```python
from build123d import *

# Parameters (mm, degrees)
F1_R     = 8.89
F1_R_2   = 5.9436
F3_R     = 8.89
F3_R_2   = 7.62
F4_DEPTH = 12.7
F5_R     = 8.89
F5_R_2   = 7.62
F6_DEPTH = 12.7


with BuildPart() as f2:
    # F2: sweep along a path in F0
    with BuildLine(Plane.XY) as f2_path:
        Line((0, 0), (0, 145.0086))
    # F1 (on Front) → F2 (sweep)
    with BuildSketch(Plane.XZ):
        Circle(F1_R)
        Circle(F1_R_2, mode=Mode.SUBTRACT)
    sweep(path=f2_path.line)

    # F3 (on face) → F4 (cut)
    with BuildSketch(Plane(origin=(0, 145.0086, 0), x_dir=(-1, 0, 0), z_dir=(0, 1, 0))):
        Circle(F3_R)
        Circle(F3_R_2, mode=Mode.SUBTRACT)
    extrude(amount=-F4_DEPTH, mode=Mode.SUBTRACT)

    # F5 (on face) → F6 (cut)
    with BuildSketch(Plane.XZ):
        Circle(F5_R)
        Circle(F5_R_2, mode=Mode.SUBTRACT)
    extrude(amount=-F6_DEPTH, mode=Mode.SUBTRACT)


solid = f2.part
```
The listing builds one solid part. Answer for the finished solid, in the listing's coordinates (mm). A direction names the side the tool comes from. Coordinates: 2 decimals unless noted, no trailing zeros. Write each loop counter-clockwise with the first axis right and the second up, starting at its lowest first coordinate (ties: lowest second). Pieces come first, ordered by that corner, then holes. Notation, with made-up numbers: (-35, 50.5) -> (-16, 50.5) arc R8 ccw to (-16, 64.5) -> close; hole circle Ø8 at (73.5, 44.25). An arc over 180 degrees is marked (long way). Write each question's results on one line, items separated by ' | '. Start each with the question number.
1) Flat-ended cylindrical pins translate along their axes: pin 1 Ø3 at (y, z) = (93.5, -4.5) entering from +X; pin 2 Ø8 at (y, z) = (18, -5.5) entering from +X; pin 3 Ø1 at (x, y) = (-5.5, 62.5) entering from -Z. Find the tip coordinate at first contact, or state that the pin passes through.
2) For a pull along X with two mould halves and no side action, classify faces 4 (the flat face through (-4, 0, 5)), 5 (the cylindrical face through (-1.93, 73.34, 8.68)), 6 (the cylindrical face through (5.669, 73.519, -1.785)) as +X half, -X half, draft (parallel to the pull), parting line (faces both ways), or undercut.
3) Straight lines are drawn through the part: probe 1 along Z at (x, y) = (0, 41.5); probe 2 along X at (y, z) = (138.5, -0.5); probe 3 along Z at (x, y) = (1.5, 33). For each, find the intervals that lie inside material, in ascending order.
4) A cutting plane is placed at B-B (z = 0). Determine the outline of the cut face in (x, y), then the cut area to 3 significant figures.
5) A cutting plane is placed at A-A (x = 0). Determine the outline of the cut face in (y, z), then the cut area to 3 significant figures.
6) A tool of negligible diameter and unlimited length cuts with its end or side. For faces 1 (the flat face through (-7, 132.309, 4)), 2 (the flat face through (-4, 145.009, 5)), 3 (the cylindrical face through (-1.65, 6.26, -7.44)), from which of +Z, -Z, +X, -X, +Y, -Y can it reach the whole face along a straight path? Write none if from no direction.
7) A cutting plane is placed at C-C (y = 130.5). Determine the outline of the cut face in (x, z), then the cut area to 3 significant figures.
Values follow:
1) pin 1: x = 8.37 | pin 2: x = 8.76 | pin 3: z = -7.35
2) face 4: draft | face 5: parting line | face 6: undercut
3) probe 1: -8.89 to -5.94, 5.94 to 8.89 | probe 2: -7.6 to -5.92, 5.92 to 7.6 | probe 3: -8.76 to -5.75, 5.75 to 8.76
4) outline: (-8.89, 12.7) -> (-7.62, 12.7) -> (-7.62, 0) -> (-5.94, 0) -> (-5.94, 145.01) -> (-7.62, 145.01) -> (-7.62, 132.31) -> (-8.89, 132.31) -> close; (5.94, 0) -> (7.62, 0) -> (7.62, 12.7) -> (8.89, 12.7) -> (8.89, 132.31) -> (7.62, 132.31) -> (7.62, 145.01) -> (5.94, 145.01) -> close | area: 790 mm²
5) outline: (0, -7.62) -> (12.7, -7.62) -> (12.7, -8.89) -> (132.31, -8.89) -> (132.31, -7.62) -> (145.01, -7.62) -> (145.01, -5.94) -> (0, -5.94) -> close; (0, 5.94) -> (145.01, 5.94) -> (145.01, 7.62) -> (132.31, 7.62) -> (132.31, 8.89) -> (12.7, 8.89) -> (12.7, 7.62) -> (0, 7.62) -> close | area: 790 mm²
6) face 1: +Y | face 2: +Z, -Z, +X, -X, +Y | face 3: -Y
7) outline: circle Ø17.78 at (0, 0); hole circle Ø11.89 at (0, 0) | area: 137 mm²
